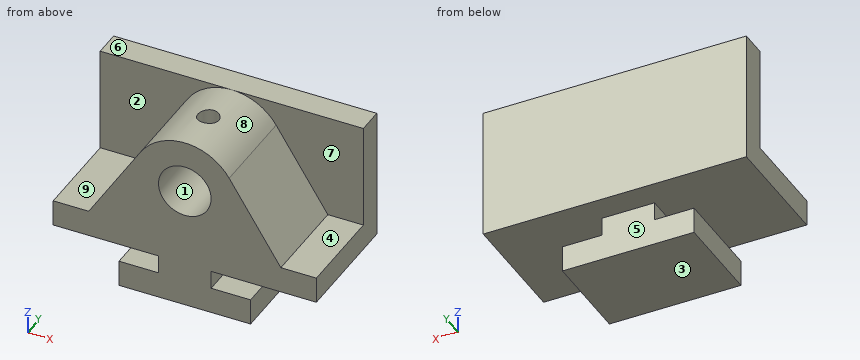
```python
from build123d import *

# Parameters (mm, degrees)
F0_R     = 12.7
F1_DEPTH = 44.45
F2_W     = 127
F2_H     = 63.5
F3_DEPTH = 12.7
F5_R     = 5.08
F6_DEPTH = 25.4


with BuildPart() as f1:
    # F0 (on Front) → F1 (new body)
    with BuildSketch(Plane.XZ):
        with BuildLine():
            Line((-31.75, 0), (0, 0))
            Line((0, 0), (31.75, 0))
            Line((31.75, 0), (31.75, 12.7))
            Line((31.75, 12.7), (12.7, 12.7))
            Line((12.7, 12.7), (12.7, 21.59))
            Line((12.7, 21.59), (63.5, 21.59))
            Line((63.5, 21.59), (63.5, 34.29))
            Line((63.5, 34.29), (46.355, 34.29))
            Line((46.355, 34.29), (21.407995, 73.359592))
            ThreePointArc((21.407995, 73.359592), (0, 85.09), (-21.407995, 73.359592))
            Line((-21.407995, 73.359592), (-46.355, 34.29))
            Line((-46.355, 34.29), (-63.5, 34.29))
            Line((-63.5, 34.29), (-63.5, 21.59))
            Line((-63.5, 21.59), (-12.7, 21.59))
            Line((-12.7, 21.59), (-12.7, 12.7))
            Line((-12.7, 12.7), (-31.75, 12.7))
            Line((-31.75, 12.7), (-31.75, 0))
        make_face()
        with Locations((0, 59.69)):
            Circle(F0_R, mode=Mode.SUBTRACT)
    extrude(amount=F1_DEPTH)

    # F2 (on face) → F3 (join)
    with BuildSketch(Plane(origin=(0, 0, 0), x_dir=(-1, 0, 0), z_dir=(0, 1, 0))):
        with Locations((0, 53.34)):
            Rectangle(F2_W, F2_H)
    extrude(amount=F3_DEPTH)

    # F5 (on offset) → F6 (cut)
    with BuildSketch(Plane.XY.offset(85.09)):
        with Locations((0, -22.225)):
            Circle(F5_R)
    extrude(amount=-F6_DEPTH, mode=Mode.SUBTRACT)


solid = f1.part
```
Input: part model. Units: mm. Frame: model coordinates. Face numbers are marked on the shaded views. A direction names the side the tool comes from. Coordinates: 2 decimals unless noted, no trailing zeros. Write each loop counter-clockwise with the first axis right and the second up, starting at its lowest first coordinate (ties: lowest second). Pieces come first, ordered by that corner, then holes.
1) Section B-B on z = 42. Output: boundary loops of the cut face in (x, y), and give its area (3 significant figures).
2) Section C-C on y = -25. Output: boundary loops of the cut face in (x, z) (3 decimals).
3) Section D-D on z = 76. Output: boundary loops of the cut face in (x, y) (3 decimals).
4) Mould query, pull axis Z, two halves, no side actions, for the marked faces 1, 2, 3 and 4. Classes: pulls with the +Z half, pulls with the -Z half, needs draft (parallel to the pull), parting line crosses it, or undercut.
5) Section A-A on y = -31. Output: boundary loops of the cut face in (x, z) (3 decimals), and give its area (3 significant figures).
6) Material intervals for line 1 along Z through (x, y) = (0, -31.5); line 2 along Y through (x, z) = (0, 80.25) (3 decimals); line 3 along Y through (x, z) = (53, 41), sorted ascending.
7) Pin query (flat end, axial travel): pin 1 Ø10 at (x, y) = (21.5, -15.5) entering from +Z; pin 2 Ø6.5 at (y, z) = (-29.5, 4.5) entering from -X; pin 3 Ø5 at (x, y) = (-54, -25) entering from +Z. Return the tip coordinate at first contact, or that it passes through.
8) Set-up query: the marked faces 5, 6, 7, 8 and 9. Return all of +Z, -Z, +X, -X, +Y, -Y with unobstructed straight access to the full face (end or side cutting, diameter ignored); none if empty.
Check result:
1. outline: (-63.5, 0) - (-41.43, 0) - (-41.43, -44.45) - (41.43, -44.45) - (41.43, 0) - (63.5, 0) - (63.5, 12.7) - (-63.5, 12.7) - close
1. area: 5,300 mm2
2. outline: (-63.5, 21.59) - (-12.7, 21.59) - (-12.7, 12.7) - (-31.75, 12.7) - (-31.75, 0) - (31.75, 0) - (31.75, 12.7) - (12.7, 12.7) - (12.7, 21.59) - (63.5, 21.59) - (63.5, 34.29) - (46.355, 34.29) - (21.408, 73.36) arc R25.4 ccw to (4.255, 84.731) - (4.255, 71.656) arc R12.7 cw (long way) to (-4.255, 71.656) - (-4.255, 84.731) arc R25.4 ccw to (-21.408, 73.36) - (-46.355, 34.29) - (-63.5, 34.29) - close
3. outline: (-63.5, 0) - (-19.472, 0) - (-19.472, -44.45) - (19.472, -44.45) - (19.472, 0) - (63.5, 0) - (63.5, 12.7) - (-63.5, 12.7) - close; hole circle Ø10.16 at (0, -22.225)
4. face 1: undercut
4. face 2: needs draft
4. face 3: pulls with the -Z half
4. face 4: pulls with the +Z half
5. outline: (-63.5, 21.59) - (-12.7, 21.59) - (-12.7, 12.7) - (-31.75, 12.7) - (-31.75, 0) - (31.75, 0) - (31.75, 12.7) - (12.7, 12.7) - (12.7, 21.59) - (63.5, 21.59) - (63.5, 34.29) - (46.355, 34.29) - (21.408, 73.36) arc R25.4 ccw to (-21.408, 73.36) - (-46.355, 34.29) - (-63.5, 34.29) - close; hole circle Ø25.4 at (0, 59.69)
5. area: 5,140 mm2
6. line 1: z = 0 to 46.99, 72.39 to 85.09
6. line 2: y = -44.45 to -27.305, -17.145 to 12.7
6. line 3: y = 0 to 12.7
7. pin 1: stops at z = 79
7. pin 2: stops at x = -31.75
7. pin 3: stops at z = 34.29
8. face 5: -Z, +X, -X, +Y
8. face 6: +Z, +X, -X, +Y, -Y
8. face 7: +Z, +X, -Y
8. face 8: +Z, -Y
8. face 9: +Z, -X, -Y
